Verification items for this drawing (mm, ordinates from the low corner). A direction names the side the tool comes from. Give positions to 0.01 mm unless a question says otherwise; leave off trailing zeros. Order: outer loops, then holes, each group sorted by start corner. A loop starts at its lowest first (then second) coordinate and runs counter-clockwise, first axis right, second up. Notation, with made-up numbers: M 63.5,11.25 L 76.5,11.25 A26 ccw 76.5,30.25 Z; hole C 73,-30.75 d9. An arc over 180 degrees is marked long. Answer as a JSON object with one key per item and string values.
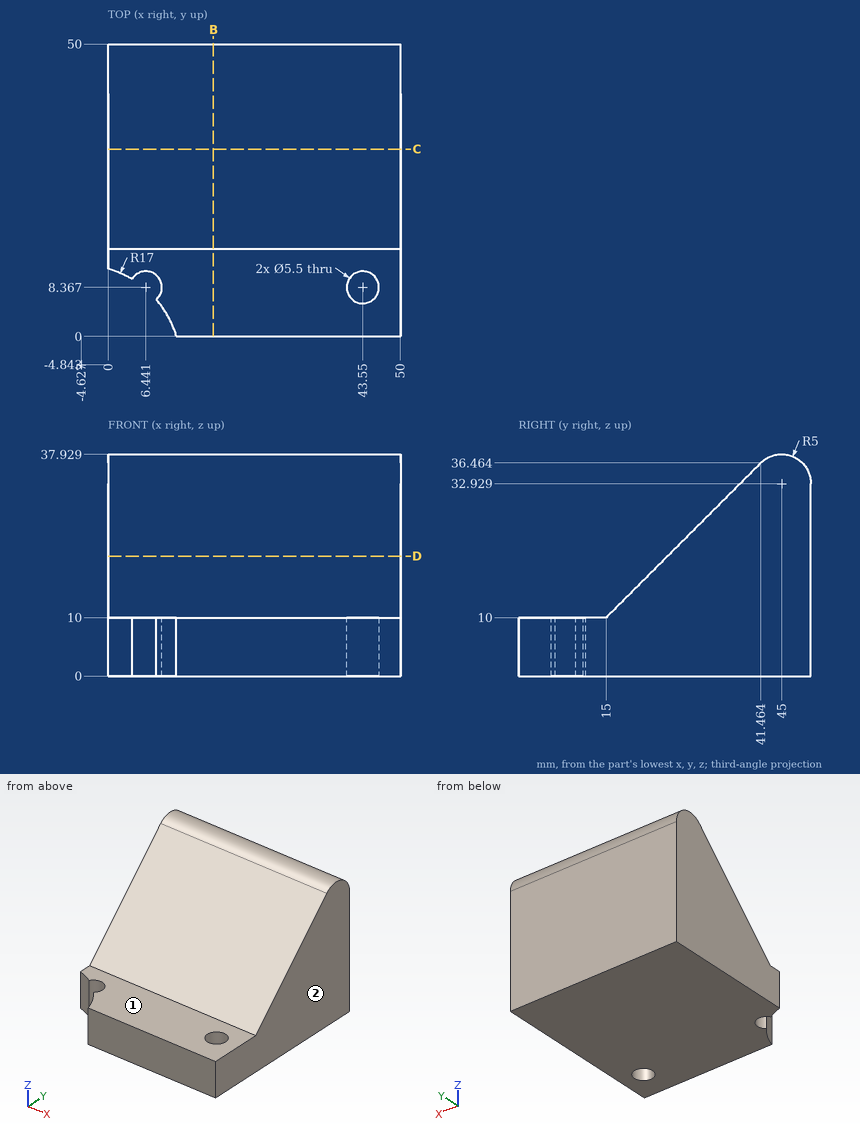
Q1. Gauge pin test, flat ends, axial feed: pin 1 Ø7.5 at (x, y) = (20, 8.5) entering from +Z; pin 2 Ø1 at (x, y) = (36.5, 43) entering from +Z. Record the tip position at first contact, or that the pin passes through.
Resolved:
{"pin 1": "stops at z = 10", "pin 2": "stops at z = 37.7"}
Q2. Section check B-B on x = 18. Record the cut outline in (y, z) (1 decimal).
Resolved:
{"outline": "M 0,0 L 50,0 L 50,32.9 A5 ccw 41.5,36.5 L 15,10 L 0,10 Z"}
Q3. Section check D-D on z = 20.5. Record the cut outline in (x, y), then the cut area to 4 significant figures.
Resolved:
{"outline": "M 0,25.5 L 50,25.5 L 50,50 L 0,50 Z", "area": "1,225 mm²"}
Q4. Section check C-C on y = 32. Record the cut outline in (x, z).
Resolved:
{"outline": "M 0,0 L 50,0 L 50,27 L 0,27 Z"}
Q5. Tool access check on the marked faces 1 and 2. Record the directions out of +Z, -Z, +X, -X, +Y, -Y that give a thin tool (end or side, any length) a straight path to the whole face; none if there is none.
Resolved:
{"face 1": "+Z, +X, -X, -Y", "face 2": "+Z, -Z, +X, +Y, -Y"}
Q6. Material ranges on L1, parallel to Z at x = 36, y = 13.5; L2, parallel to Y at x = 31, z = 21.5; L3, parallel to Z at x = 29.5, y = 23.5, recorded low to high.
Resolved:
{"L1": "z = 0 to 10", "L2": "y = 26.5 to 50", "L3": "z = 0 to 18.5"}
